Here's the drawing with two shaded views (mm, measured from the low corner). I have some questions. A direction names the side the tool comes from. Coordinates: 2 decimals unless noted, no trailing zeros. Loops run counter-clockwise (first coordinate to the right, second up) from the corner with the lowest first, then second, coordinate; pieces in that order, holes last.
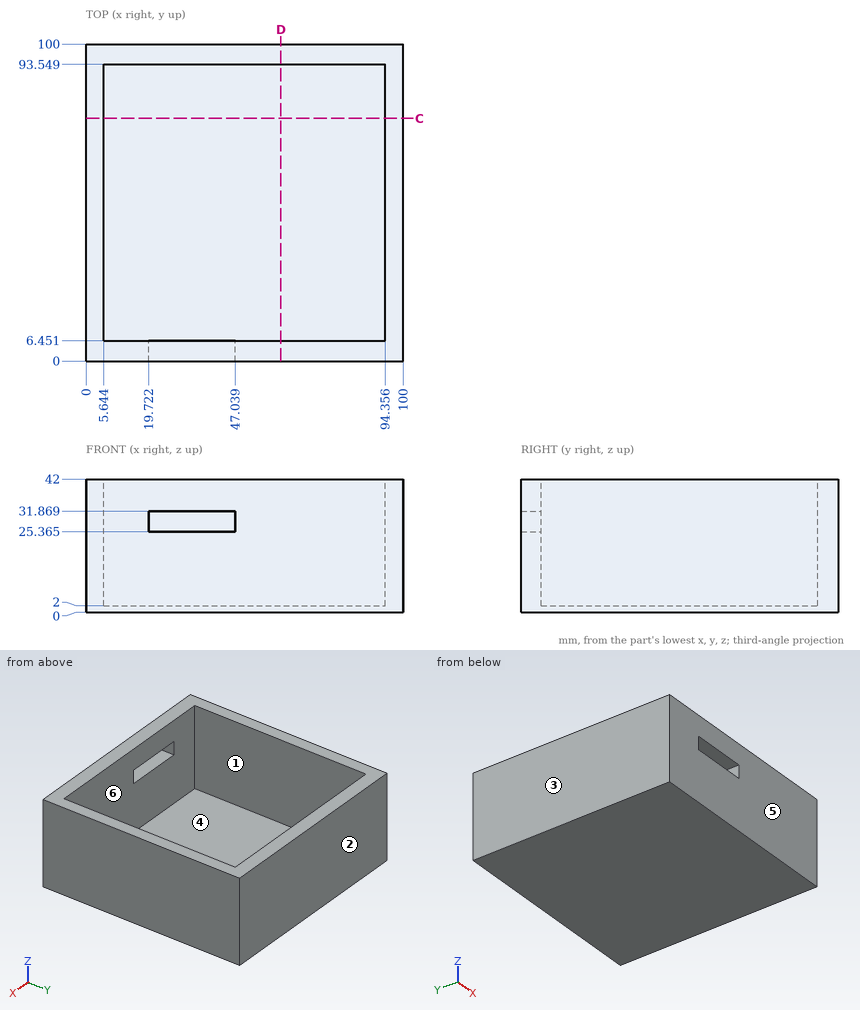
(1) If we mould it in two halves opening along X, with no side actions, what happens to the marked faces 1, 2, 3 and 4? For each: released by +X, released by -X, zero draft, split by the parting line, or undercut.
Check values:
face 1: undercut
face 2: zero draft
face 3: released by -X
face 4: undercut
(2) I want a section at C-C on y = 76.5. Write out the boundary of the cut face in (x, z) (1 decimal).
Check values:
outline: (0, 0) - (100, 0) - (100, 42) - (94.4, 42) - (94.4, 2) - (5.6, 2) - (5.6, 42) - (0, 42) - close
(3) If I drill on probe 1 along Y at (x, z) = (8, 29); probe 2 along X at (y, z) = (19.5, 20) (1 decimal); probe 3 along Y at (x, z) = (34.5, 26), over which ranges is the centre line in solid material (lowest first)?
Check values:
probe 1: y = 0 to 6.45, 93.55 to 100
probe 2: x = 0 to 5.6, 94.4 to 100
probe 3: y = 93.55 to 100
(4) Which directions (+Z, -Z, +X, -X, +Y, -Y) give clear straight access to the entire face, cutting with the end or side of a thin tool? Please do the marked faces 5 and 6.
Check values:
face 5: +Z, -Z, +X, -X, -Y
face 6: +Z
(5) I want a section at D-D on x = 61.5. Write out the boundary of the cut face in (y, z), then the cut area to 3 significant figures.
Check values:
outline: (0, 0) - (100, 0) - (100, 42) - (93.55, 42) - (93.55, 2) - (6.45, 2) - (6.45, 42) - (0, 42) - close
area: 716 mm2
